Build history of the part. All positions in model axes, mm. A direction names the side the tool comes from. Coordinates: 2 decimals unless noted, no trailing zeros. Loops run counter-clockwise (first coordinate to the right, second up) from the corner with the lowest first, then second, coordinate; pieces in that order, holes last.
Item 1: Flat gauge pins, fed straight in: pin 1 (1.5 mm diameter, centred on x = 21.5, y = 5, fed in from +Z); pin 2 (14 mm diameter, centred on x = 21.5, y = 23.5, fed in from +Z). Where does each tip first touch, or does it go through?
Item 2: Mould opens along X. For faces 3 (the face through (0, 19, 15)), 4 (the face through (25, 16, 0)), 5 (the face through (12.7, 27, 27)) say: released by +X, released by -X, zero draft, split by the parting line, or undercut.
Item 3: Cut at D-D (z = 31). List the corners of the cut face in (x, y).
Item 4: 3-axis set-ups, long thin cutter, end or side, ignore diameter. For faces 1 (the face through (38.1, 27, 27)), 2 (the face through (25, 0, 6)): which of +Z, -Z, +X, -X, +Y, -Y reach the whole face in a straight line?
Item 5: Cut at C-C (y = 27). List the corners of the cut face in (x, z).
Item 6: Cut at B-B (x = 20.5). List the corners of the cut face in (y, z), and give its area (3 significant figures).
Item 7: Cut at A-A (z = 24.5). List the corners of the cut face in (x, y).
Item 8: Drill centre lines: line 1 along X through (y, z) = (27, 34.5); line 2 along Z through (x, y) = (32, 20.5); line 3 along Y through (x, z) = (35.5, 16). Where is each one in solid material? Low to high.
from build123d import *

# Parameters (mm, degrees)
F0_W     = 50.8
F0_H     = 38.1
F1_DEPTH = 31.75
F2_W     = 25.4
F2_H     = 19.05
F3_DEPTH = 19.05
F5_DEPTH = 50.8


with BuildPart() as f1:
    # F0 (on Front) → F1 (new body)
    with BuildSketch(Plane.XZ):
        with Locations((25.4, 19.05)):
            Rectangle(F0_W, F0_H)
    extrude(amount=-F1_DEPTH)

    # F2 (on face) → F3 (cut)
    with BuildSketch(Plane.XY.offset(38.1)):
        with Locations((25.4, 22.225)):
            Rectangle(F2_W, F2_H)
    extrude(amount=-F3_DEPTH, mode=Mode.SUBTRACT)

    # F4 (on face) → F5 (cut)
    with BuildSketch(Plane.YZ.offset(50.8)):
        with BuildLine():
            Line((0, 38.1), (0, 12.7))
            ThreePointArc((0, 12.7), (16.764354, 21.335646), (25.4, 38.1))
            Line((25.4, 38.1), (0, 38.1))
        make_face()
    extrude(amount=-F5_DEPTH, mode=Mode.SUBTRACT)


solid = f1.part
Filled sheet:
1. pin 1: stops at z = 14.24
1. pin 2: stops at z = 19.05
2. face 3: released by -X
2. face 4: zero draft
2. face 5: undercut
3. outline: (0, 23.31) - (12.7, 23.31) - (12.7, 31.75) - (0, 31.75) - close; (38.1, 23.31) - (50.8, 23.31) - (50.8, 31.75) - (38.1, 31.75) - close
4. face 1: +Z, +Y, -Y
4. face 2: +Z, -Z, +X, -X, -Y
5. outline: (0, 0) - (50.8, 0) - (50.8, 38.1) - (38.1, 38.1) - (38.1, 19.05) - (12.7, 19.05) - (12.7, 38.1) - (0, 38.1) - close
6. outline: (0, 0) - (31.75, 0) - (31.75, 19.05) - (14.21, 19.05) arc R30.93 cw to (0, 12.7) - close
6. area: 549 mm2
7. outline: (0, 19.53) - (12.7, 19.53) - (12.7, 31.75) - (0, 31.75) - close; (38.1, 19.53) - (50.8, 19.53) - (50.8, 31.75) - (38.1, 31.75) - close
8. line 1: x = 0 to 12.7, 38.1 to 50.8
8. line 2: z = 0 to 19.05
8. line 3: y = 9.61 to 31.75
